The drawing under review shows one solid part. Ordinate dimensions are in mm from its lowest x, y, z. A direction names the side the tool comes from. Give positions to 0.01 mm unless a question says otherwise; leave off trailing zeros. Order: outer loops, then holes, each group sorted by start corner. A loop starts at its lowest first (then second) coordinate and runs counter-clockwise, first axis right, second up. Notation, with made-up numbers: (-6.5, 1) -> (37.5, 1) arc R24 cw to (37.5, 38) -> close; hole circle Ø1 at (12.25, 40.5). An arc over 180 degrees is marked (long way). Return JSON: item names as keys, results as strings. Group by question number.
1) The part is to be moulded in two halves that separate along X. For the marked faces 3, 4 and 5, say which applies: released by +X, released by -X, zero draft, split by the parting line, or undercut.
2) To check wall thickness, follow line 1 along Z through (x, y) = (2.25, 5.75); line 2 along X through (y, z) = (4, 4.25); line 3 along X through (y, z) = (11, 4.75). State the ranges of each line that lie inside material, in increasing order.
3) Insertion check: P1, Ø4, axis at x = 9, y = 2.5, coming from the +Z side; P2, Ø2.5, axis at x = 2.25, z = 5, coming from the +Y side (3 decimals). Each pin has a flat end and moves straight along its axis. Give the tip position at first contact, or say it passes through.
4) Add section A-A (y = 3.75). Give the boundary of the cut face in (x, z).
5) For the marked faces 1 and 2, list the 3-axis set-ups (+Z, -Z, +X, -X, +Y, -Y) from which the entire face can be reached by the end or side of a thin tool; tool diameter is ignored.
6) Add section B-B (x = 2.25). Give the boundary of the cut face in (y, z).
7) Add section D-D (y = 8.5). Give the boundary of the cut face in (x, z), then the cut area to 3 significant figures.
8) Add section C-C (z = 3.75). Give the boundary of the cut face in (x, y).
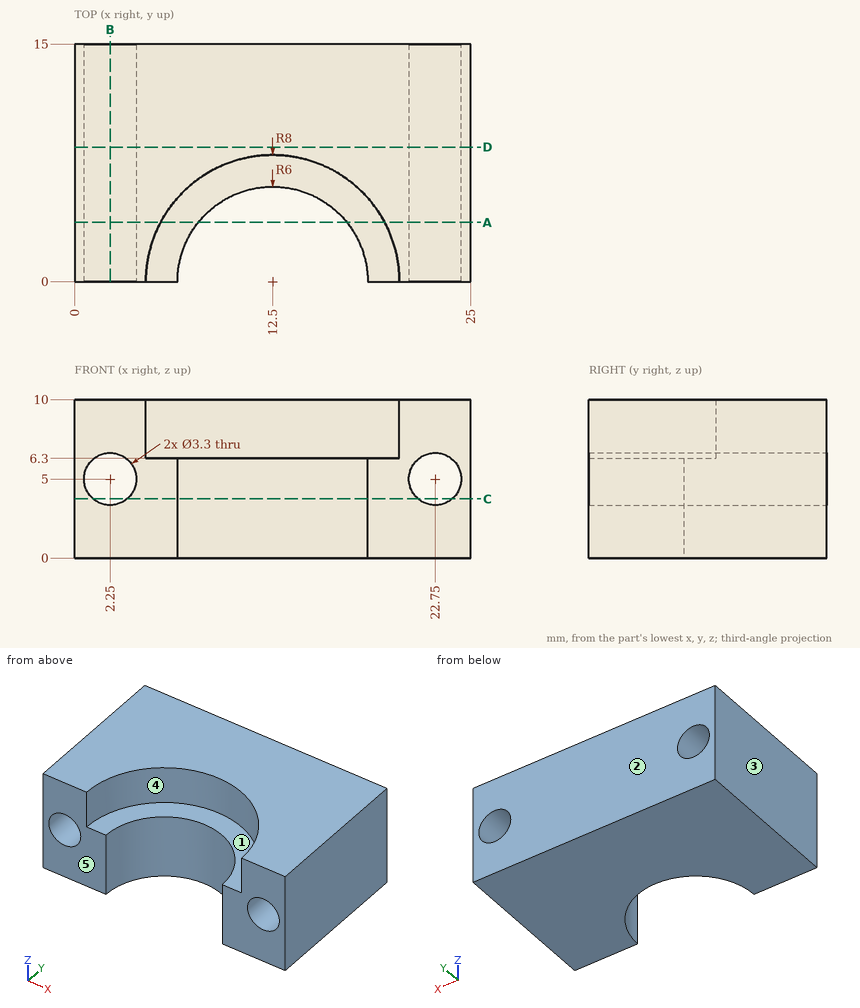
Evaluation:
{
 "1": {"face 3": "released by -X", "face 4": "undercut", "face 5": "zero draft"},
 "2": {"line 1": "0 to 3.35, 6.65 to 10", "line 2": "0 to 0.78, 3.72 to 8.03, 16.97 to 21.28, 24.22 to 25", "line 3": "0 to 0.62, 3.88 to 21.12, 24.38 to 25"},
 "3": {"P1": "z = 6.3", "P2": "through"},
 "4": {"outline": "(0, 0) -> (7.82, 0) -> (7.82, 6.3) -> (5.43, 6.3) -> (5.43, 10) -> (0, 10) -> close; (17.18, 0) -> (25, 0) -> (25, 10) -> (19.57, 10) -> (19.57, 6.3) -> (17.18, 6.3) -> close; hole circle Ø3.3 at (2.25, 5); hole circle Ø3.3 at (22.75, 5)"},
 "5": {"face 1": "+Z, -Y", "face 2": "+Z, -Z, +X, -X, +Y"},
 "6": {"outline": "(0, 0) -> (15, 0) -> (15, 3.35) -> (0, 3.35) -> close; (0, 6.65) -> (15, 6.65) -> (15, 10) -> (0, 10) -> close"},
 "7": {"outline": "(0, 0) -> (25, 0) -> (25, 10) -> (0, 10) -> close; hole circle Ø3.3 at (2.25, 5); hole circle Ø3.3 at (22.75, 5)", "area": "233 mm^2"},
 "8": {"outline": "(0, 0) -> (1.17, 0) -> (1.17, 15) -> (0, 15) -> close; (3.33, 0) -> (6.5, 0) arc R6 cw to (18.5, 0) -> (21.67, 0) -> (21.67, 15) -> (3.33, 15) -> close; (23.83, 0) -> (25, 0) -> (25, 15) -> (23.83, 15) -> close"}
}
